Here's how the part is built. I have some questions about the finished solid (model axes, mm). A direction names the side the tool comes from. Round coordinates to 2 decimals unless told otherwise and drop trailing zeros. Loops run counter-clockwise (first coordinate to the right, second up) from the corner with the lowest first, then second, coordinate; pieces in that order, holes last. Notation, with made-up numbers: M 7.5,80.5 L 42.5,80.5 A26 ccw 42.5,103.5 Z; hole C 29,72 d4. An arc over 180 degrees is marked long. Use a Markdown table: item, result.
from build123d import *

# Parameters (mm, degrees)
F0_W     = 12.1
F0_H     = 12.1
F1_DEPTH = 6
F2_R     = 2
F3_DEPTH = 5
F4_W     = 10
F4_H     = 10
F5_DEPTH = 1


with BuildPart() as f1:
    # F0 (on Top) → F1 (new body)
    with BuildSketch(Plane.XY):
        with Locations((-39.792942, 6.276945)):
            Rectangle(F0_W, F0_H)
    extrude(amount=F1_DEPTH)

    # F2 (on face) → F3 (cut)
    with BuildSketch(Plane(origin=(0, 0, 0), x_dir=(1, 0, 0), z_dir=(0, 0, -1))):
        with Locations((-39.792942, -3.251945)):
            Circle(F2_R)
        with Locations((-39.792942, -9.301945)):
            Circle(F2_R)
    extrude(amount=-F3_DEPTH, mode=Mode.SUBTRACT)

    # F4 (on face) → F5 (join)
    with BuildSketch(Plane.XY.offset(6)):
        with Locations((-39.792942, 6.276945)):
            Rectangle(F4_W, F4_H)
    extrude(amount=F5_DEPTH)


solid = f1.part
1. For pin 1 Ø0.8 at (y, z) = (4.5, 6.5) entering from +X; pin 2 Ø3 at (x, y) = (-40, 3.5) entering from -Z; pin 3 Ø0.5 at (x, z) = (-41, 6.5) entering from -Y, each with a flat end and sliding along its axis, tell me the tip position at first contact or that it passes through.
Answer sheet:
| item | result |
|---|---|
| pin 1 | x = -34.79 |
| pin 2 | z = 5 |
| pin 3 | y = 1.28 |
2. Imagine slicing it at D-D, the plane z = 6.75. Write out the boundary of the cut face in (x, y), then the cut area to 3 significant figures.
Answer sheet:
| item | result |
|---|---|
| outline | M -44.79,1.28 L -34.79,1.28 L -34.79,11.28 L -44.79,11.28 Z |
| area | 100 mm2 |
3. Imagine slicing it at B-B, the plane y = 7. Write out the boundary of the cut face in (x, z).
Answer sheet:
| item | result |
|---|---|
| outline | M -45.84,0 L -33.74,0 L -33.74,6 L -34.79,6 L -34.79,7 L -44.79,7 L -44.79,6 L -45.84,6 Z |
4. I need wall thicknesses on probe 1 along Y at (x, z) = (-40.75, 4.25); probe 2 along X at (y, z) = (9.25, 2.5); probe 3 along Y at (x, z) = (-40, 4.75). Which ranges of each line are inside material? Lowest first, please. Write a range as from..to.
Answer sheet:
| item | result |
|---|---|
| probe 1 | 0.23..1.5, 5.01..7.55, 11.06..12.33 |
| probe 2 | -45.84..-41.79, -37.79..-33.74 |
| probe 3 | 0.23..1.26, 5.24..7.31, 11.29..12.33 |
5. Imagine slicing it at C-C, the plane z = 2. Write out the boundary of the cut face in (x, y).
Answer sheet:
| item | result |
|---|---|
| outline | M -45.84,0.23 L -33.74,0.23 L -33.74,12.33 L -45.84,12.33 Z; hole C -39.79,3.25 d4; hole C -39.79,9.3 d4 |
6. Which directions (+Z, -Z, +X, -X, +Y, -Y) give clear straight access to the entire face, cutting with the end or side of a thin tool? Please do faces 5 (the face through (-39.9, 1.277, 6.5)), 6 (the face through (-39.9, 11.277, 6.5)), 7 (the face through (-34.793, 6.2, 6.5)), 8 (the face through (-40, 3, 5)).
Answer sheet:
| item | result |
|---|---|
| face 5 | +Z, +X, -X, -Y |
| face 6 | +Z, +X, -X, +Y |
| face 7 | +Z, +X, +Y, -Y |
| face 8 | -Z |
7. Imagine slicing it at A-A, the plane x = -42.5. Write out the boundary of the cut face in (y, z), then the cut area to 3 significant figures.
Answer sheet:
| item | result |
|---|---|
| outline | M 0.23,0 L 12.33,0 L 12.33,6 L 11.28,6 L 11.28,7 L 1.28,7 L 1.28,6 L 0.23,6 Z |
| area | 82.6 mm2 |
8. We'd pull the mould along X, two halves only. Please class faces 1 (the face through (-41.79, 9.21, 2.46)), 2 (the face through (-40, 9, 5)), 3 (the face through (-40, 12.327, 3)), 4 (the face through (-44.793, 6.2, 6.5)): +X half, -X half, draft (parallel to the pull), parting line (faces both ways), or undercut.
Answer sheet:
| item | result |
|---|---|
| face 1 | undercut |
| face 2 | undercut |
| face 3 | draft |
| face 4 | -X half |
